Job drawing, mm, ordinate dimensions from the low corner. One solid piece. A direction names the side the tool comes from. Coordinates: 2 decimals unless noted, no trailing zeros. Order: outer loops, then holes, each group sorted by start corner. A loop starts at its lowest first (then second) coordinate and runs counter-clockwise, first axis right, second up. Notation, with made-up numbers: (-37, 64.5) -> (-2, 64.5) arc R16 cw to (-2, 75.5) -> close; hole circle Ø10 at (8, 5). An arc over 180 degrees is marked (long way). Use CSV: the item, a comma, the result in double quotes. Start each with the question number.
(1) Tool access for the marked faces 1, 2, 3 and 4: list every direction of +Z, -Z, +X, -X, +Y, -Y with a clear straight run to the whole face (end or side of a thin tool).
(2) Cut at D-D on y = 17.5. Write the cut outline in (x, z).
(3) Probe L1, parallel to Z at x = 8.5, y = 7; L2, parallel to X at y = 27, z = 3; L3, parallel to X at y = 34.5, z = 20. List the from-to ranges inside material, lowest first.
(4) Cut at C-C on x = 36. Write the cut outline in (y, z), plus the area to 3 significant figures.
(5) Cut at B-B on y = 26. Write the cut outline in (x, z).
(6) Pin check, flat tips, straight feed: pin 1 Ø8 at (y, z) = (15, 31.5) entering from +X; pin 2 Ø1 at (x, y) = (6, 7.5) entering from +Z; pin 3 Ø12 at (y, z) = (17.5, 13.5) entering from -X. Stop position of each tip, or through.
(7) Cut at A-A on z = 36.5. Write the cut outline in (x, y), plus the area to 3 significant figures.
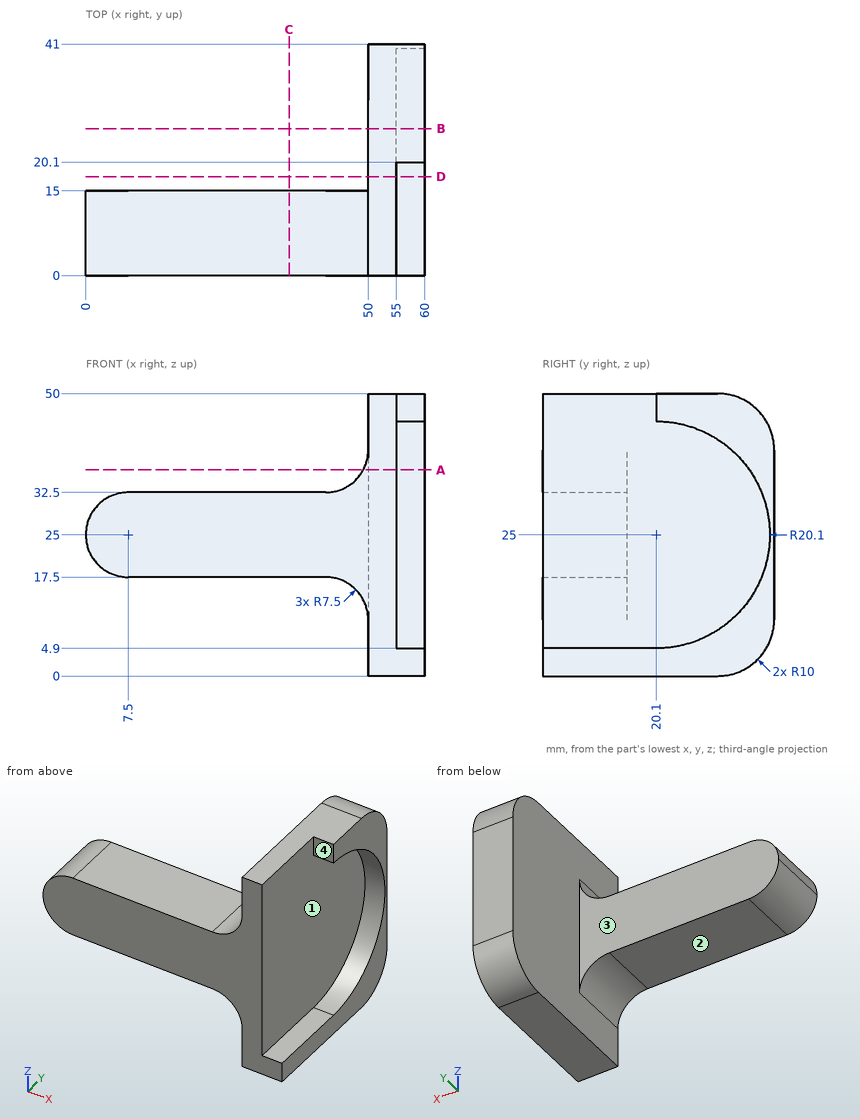
Outcome:
1,face 1,"+X, -Y"
1,face 2,"-Z, -X, +Y, -Y"
1,face 3,"+Z, -Z, -X, +Y"
1,face 4,"+Z, +X, -Y"
2,outline,"(50, 0) -> (60, 0) -> (60, 4.9) -> (55, 4.9) -> (55, 50) -> (50, 50) -> close"
3,L1,"17.5 to 32.5"
3,L2,"50 to 60"
3,L3,"50 to 55"
4,outline,"(0, 17.5) -> (15, 17.5) -> (15, 32.5) -> (0, 32.5) -> close"
4,area,"225 mm2"
5,outline,"(50, 0) -> (60, 0) -> (60, 5.79) -> (55, 5.79) -> (55, 44.21) -> (60, 44.21) -> (60, 50) -> (50, 50) -> close"
6,pin 1,"x = 55"
6,pin 2,"z = 32.43"
6,pin 3,"x = 3.06"
7,outline,"(49.13, 0) -> (55, 0) -> (55, 36.59) -> (60, 36.59) -> (60, 41) -> (50, 41) -> (50, 15) -> (49.13, 15) -> close"
7,area,"240 mm2"
